```python
from build123d import *

# Parameters (mm, degrees)
F0_W     = 1599.946
F0_H     = 1439.926
F1_DEPTH = 101.6
F3_DEPTH = 1599.947
F4_SIZE  = 25.4
F5_R     = 84.963
F6_DEPTH = 101.601


with BuildPart() as f1:
    # F0 (on Top) → F1 (new body)
    with BuildSketch(Plane.XY):
        with Locations((799.973, 719.963)):
            Rectangle(F0_W, F0_H)
    extrude(amount=-F1_DEPTH)

    # F2 (on face) → F3 (cut, through all)
    with BuildSketch(Plane.YZ.offset(1599.946)):
        Polygon((91.9988, 0), (68.0212, 0), (68.0212, -26.9914), (68.0212, -27), (59.01, -27), (59.01, -45), (101.01, -45), (101.01, -27), (91.9988, -27), (91.9988, -26.9914), align=None)
        Polygon((1371.9048, -26.9914), (1371.9048, 0), (1347.9272, 0), (1347.9272, -26.9914), (1347.9272, -27), (1338.916, -27), (1338.916, -45), (1380.916, -45), (1380.916, -27), (1371.9048, -27), align=None)
        Polygon((261.03, -27), (252.0188, -27), (252.0188, -26.9914), (252.0188, 0), (228.0412, 0), (228.0412, -26.9914), (228.0412, -27), (219.03, -27), (219.03, -45), (261.03, -45), align=None)
        Polygon((421.05, -27), (412.0388, -27), (412.0388, -26.9914), (412.0388, 0), (388.0612, 0), (388.0612, -26.9914), (388.0612, -27), (379.05, -27), (379.05, -45), (421.05, -45), align=None)
        Polygon((581.07, -27), (572.0588, -27), (572.0588, -26.9914), (572.0588, 0), (548.0812, 0), (548.0812, -26.9914), (548.0812, -27), (539.07, -27), (539.07, -45), (581.07, -45), align=None)
        Polygon((741.09, -27), (732.0788, -27), (732.0788, -26.9914), (732.0788, 0), (708.1012, 0), (708.1012, -26.9914), (708.1012, -27), (699.09, -27), (699.09, -45), (741.09, -45), align=None)
        Polygon((901.11, -27), (892.0988, -27), (892.0988, -26.9914), (892.0988, 0), (868.1212, 0), (868.1212, -26.9914), (868.1212, -27), (859.11, -27), (859.11, -45), (901.11, -45), align=None)
        Polygon((1061.13, -27), (1052.1188, -27), (1052.1188, -26.9914), (1052.1188, 0), (1028.1412, 0), (1028.1412, -26.9914), (1028.1412, -27), (1019.13, -27), (1019.13, -45), (1061.13, -45), align=None)
        Polygon((1221.15, -27), (1212.1388, -27), (1212.1388, -26.9914), (1212.1388, 0), (1188.1612, 0), (1188.1612, -26.9914), (1188.1612, -27), (1179.15, -27), (1179.15, -45), (1221.15, -45), align=None)
    extrude(amount=-F3_DEPTH, mode=Mode.SUBTRACT)

    # F4
    f4_edges = [f1.edges().sort_by_distance(p)[0] for p in [
        (1599.946, 0, -50.8),
        (1599.946, 1439.926, -50.8),
        (0, 0, -50.8),
        (0, 1439.926, -50.8),
    ]]
    chamfer(f4_edges, length=F4_SIZE)

    # F5 (on face) → F6 (cut, through all)
    with BuildSketch(Plane.XY):
        with Locations((800.1, 720.09)):
            Circle(F5_R)
    extrude(amount=-F6_DEPTH, mode=Mode.SUBTRACT)


solid = f1.part
```
Can you work these out from the model? Positions are in its coordinate system, mm. A direction names the side the tool comes from. Round coordinates to 2 decimals unless told otherwise and drop trailing zeros. Order: outer loops, then holes, each group sorted by start corner. A loop starts at its lowest first (then second) coordinate and runs counter-clockwise, first axis right, second up.
(1) If I drill on L1, parallel to Y at x = 800.1, z = -50; L2, parallel to X at y = 720.09, z = -79; L3, parallel to Z at x = 698, y = 67, over which ranges is the centre line in solid material (lowest first)?
Results are:
L1: y = 0 to 635.13, 805.05 to 1439.93
L2: x = 0 to 715.14, 885.06 to 1599.95
L3: z = -101.6 to -45, -27 to 0
(2) We'd pull the mould along Y, two halves only. Please class faces 1 (the face through (789, 161, 0)), 2 (the face through (811, 240, -45)), 3 (the face through (789, 1439.926, -50)), 4 (the face through (789, 0, -50)): +Y half, -Y half, draft (parallel to the pull), parting line (faces both ways), or undercut.
Results are:
face 1: draft
face 2: undercut
face 3: +Y half
face 4: -Y half
(3) I'm going to push a flat-ended pin straight in: pin 1 (6 mm diameter, centred on x = 857.5, y = 881.5, fed in from +Z). Where does the tip first touch, or does it pass through?
Results are:
pin 1: stops at z = -45
(4) On a 3-axis mill with a long thin cutter (end or side, diameter ignored), from which of +Z, -Z, +X, -X, +Y, -Y can I reach the whole of each face in a straight line? I mean faces 5 (the face through (789, 816, 0)), 6 (the face through (811, 1200, -45)). Say none if no direction works.
Results are:
face 5: +Z, +X, -X, +Y, -Y
face 6: +X, -X
(5) If we section it at A-A (y = 664): Please give me the cut outline in (x, z), plus the area to 3 significant figures.
Results are:
outline: (0, -101.6) - (736.28, -101.6) - (736.28, 0) - (0, 0) - close; (863.92, -101.6) - (1599.95, -101.6) - (1599.95, 0) - (863.92, 0) - close
area: 150,000 mm2
